from build123d import *

# Parameters (mm, degrees)
F0_R     = 62.635171
F1_DEPTH = 12.7
F3_DEPTH = 12.7


with BuildPart() as f1:
    # F0 (on Top) → F1 (new body, symmetric)
    with BuildSketch(Plane.XY):
        Circle(F0_R)
    extrude(amount=F1_DEPTH, both=True)

    # F2 (on face) → F3 (cut, symmetric)
    with BuildSketch(Plane.XY.offset(12.7)):
        with BuildLine():
            ThreePointArc((-62.084642, 8.286243), (-41.587534, 46.836328), (-0.88331, 62.628942))
            ThreePointArc((-0.88331, 62.628942), (-54.933436, 61.866626), (-62.084642, 8.286243))
        make_face()
        with BuildLine():
            ThreePointArc((-62.084642, 8.286243), (-15.650946, -8.711081), (13.901029, 30.933313))
            ThreePointArc((13.901029, 30.933313), (10.023188, 48.420377), (-0.88331, 62.628942))
            ThreePointArc((-0.88331, 62.628942), (-41.587534, 46.836328), (-62.084642, 8.286243))
        make_face()
    extrude(amount=F3_DEPTH, both=True, mode=Mode.SUBTRACT)


solid = f1.part
CAD build for the part. Positions are in the model's coordinates, mm. Give positions to 0.01 mm unless a question says otherwise; leave off trailing zeros. Loops run counter-clockwise (first coordinate to the right, second up) from the corner with the lowest first, then second, coordinate; pieces in that order, holes last. Notation, with made-up numbers: M -16.75,46.5 L 3.25,46.5 A24 ccw 3.25,60.5 Z; hole C 24,76.5 d4. An arc over 180 degrees is marked long. Write each question's results on one line, items separated by ' | '.
Q1. Band-saw the part on D-D on x = -36. Write the cut outline in (y, z).
Geometry check:
outline: M -51.26,-12.7 L 51.26,-12.7 L 51.26,0 L -9.54,0 L -9.54,12.7 L -51.26,12.7 Z
Q2. Probe probe 1 along Z at (x, y) = (8.5, 43); probe 2 along X at (y, z) = (-57, 1.75); probe 3 along Y at (x, z) = (-14, 10.5). List the from-to ranges inside material, lowest first.
Geometry check:
probe 1: z = -12.7 to 0 | probe 2: x = -25.96 to 25.96 | probe 3: y = -61.05 to -8.18
Q3. Flat gauge pins, fed straight in: P1, Ø4, axis at y = -50, z = 7, coming from the -X side; P2, Ø5, axis at x = 22.5, z = -4, coming from the -Y side; P3, Ø1.5, axis at y = -4.5, z = 8.5, coming from the +X side. Where does each tip first touch, or does it go through?
Geometry check:
P1: stops at x = -40.24 | P2: stops at y = -59.36 | P3: stops at x = 62.52
Q4. Band-saw the part on C-C on y = 0. Write the cut outline in (x, z).
Geometry check:
outline: M -62.64,-12.7 L 62.64,-12.7 L 62.64,12.7 L 0,12.7 L 0,0 L -54.93,0 L -54.93,12.7 L -62.64,12.7 Z
Q5. Band-saw the part on B-B on z = 10. Write the cut outline in (x, y).
Geometry check:
outline: M -62.08,8.29 A62.64 ccw long -0.88,62.63 A41.37 cw 13.9,30.93 A41.37 cw Z
Q6. Mould opens along Y. For faces 1 (the face through (-25, 27, 0)), 2 (the face through (-1, 1, -12.7)), 3 (the face through (28.9, -55.57, 0.18)) say: pulls with the +Y half, pulls with the -Y half, needs draft (parallel to the pull), parting line crosses it, or undercut.
Geometry check:
face 1: undercut | face 2: needs draft | face 3: parting line crosses it
Q7. Band-saw the part on A-A on x = -10. Write the cut outline in (y, z), and give its area (3 significant figures).
Geometry check:
outline: M -61.83,-12.7 L 61.83,-12.7 L 61.83,0 L -6.57,0 L -6.57,12.7 L -61.83,12.7 Z | area: 2,270 mm²
